Input: part model. Units: mm. Frame: model coordinates. Face numbers are marked on the shaded views. Round coordinates to 2 decimals unless told otherwise and drop trailing zeros. Loops run counter-clockwise (first coordinate to the right, second up) from the corner with the lowest first, then second, coordinate; pieces in that order, holes last. Notation, with made-up numbers: (-13.75, 68) -> (4.25, 68) arc R19 ccw to (4.25, 95) -> close; hole circle Ø1 at (74.25, 46). An arc over 180 degrees is marked (long way). Answer as a JSON object with one key per item and string values.
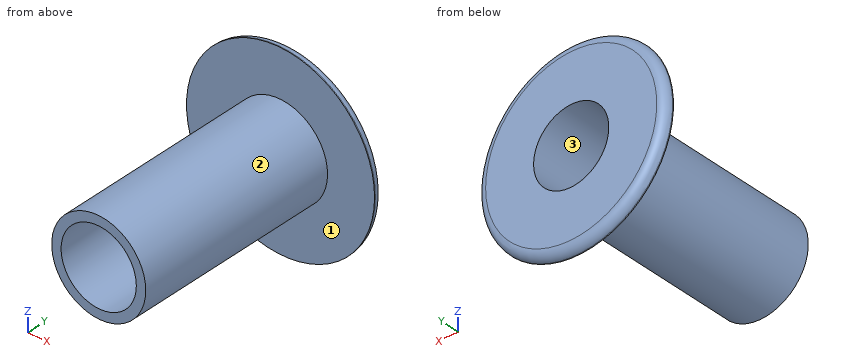
```python
from build123d import *

# Parameters (mm, degrees)
SKETCH1_R           = 1.25
SKETCH1_R_2         = 1
BOSS_EXTRUDE1_DEPTH = 5.5
SKETCH2_R           = 2.5
SKETCH2_R_2         = 1
BOSS_EXTRUDE2_DEPTH = 0.25
FILLET1_R           = 0.225


with BuildPart() as part:
    # Sketch1 → Boss-Extrude1 (new body)
    with BuildSketch(Plane(origin=(0, 0, 0), x_dir=(1, 0, 0), z_dir=(0, 1, 0))):
        Circle(SKETCH1_R)
        Circle(SKETCH1_R_2, mode=Mode.SUBTRACT)
    extrude(amount=BOSS_EXTRUDE1_DEPTH)

    # Sketch2 → Boss-Extrude2 (add)
    with BuildSketch(Plane(origin=(0, 5.5, 0), x_dir=(1, 0, 0), z_dir=(0, 1, 0))):
        Circle(SKETCH2_R)
        Circle(SKETCH2_R_2, mode=Mode.SUBTRACT)
    extrude(amount=BOSS_EXTRUDE2_DEPTH)

    # Fillet1
    fillet1_edges = [part.edges().sort_by_distance(p)[0] for p in [
        (-2.5, 5.75, 0),
    ]]
    fillet(fillet1_edges, radius=FILLET1_R)


solid = part.part
```
1) Section B-B, the plane z = 0. Output: boundary loops of the cut face in (x, y) (3 decimals).
Output:
{"outline": "(-2.5, 5.5) -> (-1.25, 5.5) -> (-1.25, 0) -> (-1, 0) -> (-1, 5.75) -> (-2.275, 5.75) arc R0.225 ccw to (-2.5, 5.525) -> close; (1, 0) -> (1.25, 0) -> (1.25, 5.5) -> (2.5, 5.5) -> (2.5, 5.525) arc R0.225 ccw to (2.275, 5.75) -> (1, 5.75) -> close"}
2) Ray query, probe 1 along Z at (x, y) = (0, 2.75); probe 2 along Y at (x, z) = (1.35, -0.5). Return the intervals inside material, ascending.
Output:
{"probe 1": "z = -1.25 to -1, 1 to 1.25", "probe 2": "y = 5.5 to 5.75"}
3) Section A-A, the plane x = 0. Output: boundary loops of the cut face in (y, z) (3 decimals).
Output:
{"outline": "(0, -1.25) -> (5.5, -1.25) -> (5.5, -2.5) -> (5.525, -2.5) arc R0.225 ccw to (5.75, -2.275) -> (5.75, -1) -> (0, -1) -> close; (0, 1) -> (5.75, 1) -> (5.75, 2.275) arc R0.225 ccw to (5.525, 2.5) -> (5.5, 2.5) -> (5.5, 1.25) -> (0, 1.25) -> close"}
4) Section C-C, the plane y = 4.95. Output: boundary loops of the cut face in (x, z).
Output:
{"outline": "circle Ø2.5 at (0, 0); hole circle Ø2 at (0, 0)"}
5) Contact query for flat-ended pins moving along their axis: P1, Ø3, axis at x = 1.5, y = 3.5, coming from the -Z side; P2, Ø1, axis at x = -1, z = -1.5, coming from the -Y side; P3, Ø2, axis at y = 3, z = 1, coming from the +X side. Output: stop coordinate, or through.
Output:
{"P1": "stops at z = -1.25", "P2": "stops at y = 5.5", "P3": "stops at x = 1.25"}
6) Draft query along Z for the marked faces 1, 2 and 3. Return one class per face: +Z half, -Z half, draft (parallel to the pull), parting line (faces both ways), or undercut.
Output:
{"face 1": "draft", "face 2": "parting line", "face 3": "undercut"}
